Design review of the part built by this model. Coordinates are the model's own, in mm. A direction names the side the tool comes from. Give positions to 0.01 mm unless a question says otherwise; leave off trailing zeros. Write each loop counter-clockwise with the first axis right and the second up, starting at its lowest first coordinate (ties: lowest second). Pieces come first, ordered by that corner, then holes. Notation, with made-up numbers: (-1, 59.5) -> (34, 59.5) arc R15 ccw to (34, 71.5) -> close; hole circle Ø8 at (73, -6). An arc over 180 degrees is marked (long way). Write each question's results on one line, items separated by ' | '. Start each with the question number.
(1) Take a section at C-C (y = 2.5). State the section outline as (x, z) points (1 decimal), plus the area to 3 significant figures.
(2) To check wall thickness, follow probe 1 along Z at (x, y) = (-1.5, 0.5) (3 decimals); probe 2 along X at (y, z) = (3, -0.25); probe 3 along X at (y, z) = (1.5, -0.75). State the ranges of each line that lie inside material, in increasing order.
(3) Mouldability with a two-part tool opening along X and no side actions: class faces 3 (the face through (6.35, 9, 0)), 4 (the face through (-7.461, 1.565, 1.514)), 5 (the face through (0, 0, 1)) as released by +X, released by -X, zero draft, split by the parting line, or undercut.
(4) For faces 1 (the face through (-5, 3.175, 0)), 2 (the face through (3, 3, 3.175)), list the 3-axis set-ups (+Z, -Z, +X, -X, +Y, -Y) from which the entire face can be reached by the end or side of a thin tool; tool diameter is ignored.
(5) Take a section at B-B (z = -1.25). Count the separate pieces of the cut face and the enclosed holes in it, plus the area to 3 significant figures.
(6) Take a section at D-D (x = -5.5). State the section outline as (y, z) points (3 decimals), plus the area to 3 significant figures.
(7) Clearance check with a flat-ended pin moving along its axis: pin 1 (3.5 mm diameter, centred on x = -1.59, z = 0, fed in from +Y) (3 decimals). State where the tip first meets the part, or that it passes through.
from build123d import *

# Parameters (mm, degrees)
SKETCH1_W           = 20.6375
SKETCH1_H           = 6.35
SKETCH1_R           = 1.5875
BOSS_EXTRUDE1_DEPTH = 3.175
SKETCH1_3_W         = 7.9375
SKETCH1_3_H         = 6.35
BOSS_EXTRUDE2_DEPTH = 9.525
FILLET1_R           = 2.38125
CUT_EXTRUDE1_DEPTH  = 31.287569645


with BuildPart() as part:
    # Sketch1 → Boss-Extrude1 (new body)
    with BuildSketch(Plane(origin=(0, 0, 0), x_dir=(1, 0, 0), z_dir=(0, 1, 0))):
        with Locations((-3.96875, 0)):
            Rectangle(SKETCH1_W, SKETCH1_H)
        with Locations(Location((-7.9375, 0, 0), (0, 0, 270))):
            Circle(SKETCH1_R, mode=Mode.SUBTRACT)
        with Locations(Location((-1.5875, 0, 0), (0, 0, 270))):
            Circle(SKETCH1_R, mode=Mode.SUBTRACT)
    extrude(amount=BOSS_EXTRUDE1_DEPTH)

    # Sketch1_3 → Boss-Extrude2 (add)
    with BuildSketch(Plane(origin=(0, 0, 0), x_dir=(1, 0, 0), z_dir=(0, 1, 0))):
        with Locations((10.31875, 0)):
            Rectangle(SKETCH1_3_W, SKETCH1_3_H)
    extrude(amount=BOSS_EXTRUDE2_DEPTH)

    # Fillet1
    fillet1_edges = [part.edges().sort_by_distance(p)[0] for p in [
        (6.35, 3.175, 0),
    ]]
    fillet(fillet1_edges, radius=FILLET1_R)

    # Sketch2 → Cut-Extrude1 (cut, through all)
    with BuildSketch(Plane(origin=(14.2875, 0, 0), x_dir=(0, 0, -1), z_dir=(1, 0, 0))):
        with BuildLine():
            ThreePointArc((0, 8.73125), (-2.38125, 6.35), (0, 3.96875))
            Line((0, 3.96875), (0, 8.73125))
        make_face()
        with BuildLine():
            Line((0, 8.73125), (0, 3.96875))
            ThreePointArc((0, 3.96875), (1.683798023, 4.666201977), (2.38125, 6.35))
            ThreePointArc((2.38125, 6.35), (1.683798023, 8.033798023), (0, 8.73125))
        make_face()
    extrude(amount=-CUT_EXTRUDE1_DEPTH, mode=Mode.SUBTRACT)


solid = part.part
Report:
1) outline: (-14.3, -3.2) -> (14.3, -3.2) -> (14.3, 3.2) -> (-14.3, 3.2) -> close; hole circle Ø3.2 at (-7.9, 0); hole circle Ø3.2 at (-1.6, 0) | area: 166 mm2
2) probe 1: -3.175 to -1.585, 1.585 to 3.175 | probe 2: -14.29 to -9.51, -6.37 to -3.16, -0.02 to 14.29 | probe 3: -14.29 to -9.34, -6.54 to -2.99, -0.19 to 14.29
3) face 3: released by -X | face 4: undercut | face 5: zero draft
4) face 1: +Z, -Z, -X, +Y | face 2: +Z, +X, -X, +Y, -Y
5) separate pieces: 4 | enclosed holes: 0 | area: 97.6 mm2
6) outline: (0, -3.175) -> (3.175, -3.175) -> (3.175, 3.175) -> (0, 3.175) -> close | area: 20.2 mm2
7) pin 1: y = 3.175
